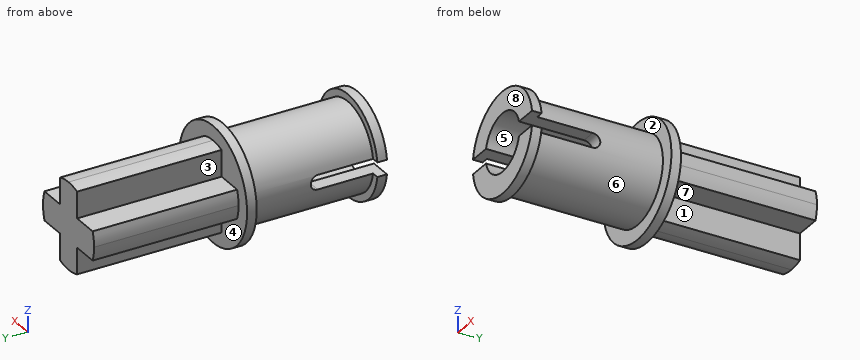
from build123d import *

# Parameters (mm, degrees)
SKETCH1_R               = 1.5
SKETCH1_R_2             = 1
BOSS_EXTRUDE1_DEPTH     = 5
SKETCH2_R               = 2
SKETCH2_R_2             = 1.5
SKETCH2_R_3             = 1
BOSS_EXTRUDE2_DEPTH     = 0.333333333
SKETCH3_R               = 1.75
SKETCH3_R_2             = 1
BOSS_EXTRUDE4_DEPTH     = 0.333333333
SKETCH4_R               = 0.25
SKETCH4_W               = 0.5
SKETCH4_H               = 2.25
CUT_EXTRUDE1_DEPTH      = 6.744562647
CUT_EXTRUDE1_DEPTH_BACK = 6.744562647
SKETCH7_W               = 1
SKETCH7_H               = 1
BOSS_EXTRUDE6_DEPTH     = 5


with BuildPart() as part:
    # Sketch1 → Boss-Extrude1 (new body)
    with BuildSketch(Plane(origin=(0, 0, 0), x_dir=(1, 0, 0), z_dir=(0, 1, 0))):
        with Locations(Location((0, 0, 0), (0, 0, 270))):
            Circle(SKETCH1_R)
        with Locations(Location((0, 0, 0), (0, 0, 270))):
            Circle(SKETCH1_R_2, mode=Mode.SUBTRACT)
    extrude(amount=BOSS_EXTRUDE1_DEPTH)

    # Sketch2 → Boss-Extrude2 (add)
    with BuildSketch(Plane(origin=(0, 5, 0), x_dir=(1, 0, 0), z_dir=(0, 1, 0))):
        with Locations(Location((0, 0, 0), (0, 0, 270))):
            Circle(SKETCH2_R)
        with Locations(Location((0, 0, 0), (0, 0, 270))):
            Circle(SKETCH2_R_2, mode=Mode.SUBTRACT)
        with Locations(Location((0, 0, 0), (0, 0, 270))):
            Circle(SKETCH2_R_2)
        with Locations(Location((0, 0, 0), (0, 0, 270))):
            Circle(SKETCH2_R_3, mode=Mode.SUBTRACT)
        with Locations(Location((0, 0, 0), (0, 0, 270))):
            Circle(SKETCH2_R_3)
    extrude(amount=-BOSS_EXTRUDE2_DEPTH)

    # Sketch3 → Boss-Extrude4 (add)
    with BuildSketch(Plane(origin=(0, 0, 0), x_dir=(-1, 0, 0), z_dir=(0, -1, 0))):
        with Locations(Location((0, 0, 0), (0, 0, 90))):
            Circle(SKETCH3_R)
        with Locations(Location((0, 0, 0), (0, 0, 270))):
            Circle(SKETCH3_R_2, mode=Mode.SUBTRACT)
    extrude(amount=-BOSS_EXTRUDE4_DEPTH)

    # Sketch4 → Cut-Extrude1 (cut, two sides)
    with BuildSketch(Plane(origin=(0, 0, 0), x_dir=(0, 0, -1), z_dir=(1, 0, 0))) as cut_extrude1_sk:
        with Locations((0, 2.25)):
            Circle(SKETCH4_R)
        with Locations((0, 1.125)):
            Rectangle(SKETCH4_W, SKETCH4_H)
    extrude(amount=CUT_EXTRUDE1_DEPTH, mode=Mode.SUBTRACT)
    extrude(cut_extrude1_sk.sketch, amount=-CUT_EXTRUDE1_DEPTH_BACK, mode=Mode.SUBTRACT)

    # Sketch7 → Boss-Extrude6 (add)
    with BuildSketch(Plane(origin=(0, 5, 0), x_dir=(1, 0, 0), z_dir=(0, 1, 0))):
        with BuildLine():
            Line((1.414213562, 0.5), (0.5, 0.5))
            Line((0.5, 0.5), (0.5, -0.5))
            Line((0.5, -0.5), (1.414213562, -0.5))
            ThreePointArc((1.414213562, -0.5), (1.478397839, -0.253652968), (1.5, 0))
            ThreePointArc((1.5, 0), (1.478397839, 0.253652968), (1.414213562, 0.5))
        make_face()
        Rectangle(SKETCH7_W, SKETCH7_H)
        with BuildLine():
            Line((0.5, -0.5), (-0.5, -0.5))
            Line((-0.5, -0.5), (-0.5, -1.414213562))
            ThreePointArc((-0.5, -1.414213562), (-0.253652968, -1.478397839), (0, -1.5))
            ThreePointArc((0, -1.5), (0.253652968, -1.478397839), (0.5, -1.414213562))
            Line((0.5, -1.414213562), (0.5, -0.5))
        make_face()
        with BuildLine():
            ThreePointArc((0.5, 1.414213562), (0.253652968, 1.478397839), (0, 1.5))
            ThreePointArc((0, 1.5), (-0.253652968, 1.478397839), (-0.5, 1.414213562))
            Line((-0.5, 1.414213562), (-0.5, 0.5))
            Line((-0.5, 0.5), (0.5, 0.5))
            Line((0.5, 0.5), (0.5, 1.414213562))
        make_face()
        with BuildLine():
            Line((-0.5, -0.5), (-0.5, 0.5))
            Line((-0.5, 0.5), (-1.414213562, 0.5))
            ThreePointArc((-1.414213562, 0.5), (-1.478397839, 0.253652968), (-1.5, 0))
            ThreePointArc((-1.5, 0), (-1.478397839, -0.253652968), (-1.414213562, -0.5))
            Line((-1.414213562, -0.5), (-0.5, -0.5))
        make_face()
    extrude(amount=BOSS_EXTRUDE6_DEPTH)


solid = part.part
Can you work these out from the model? Positions are in its coordinate system, mm. Face numbers are marked on the shaded views. A direction names the side the tool comes from. Give positions to 0.01 mm unless a question says otherwise; leave off trailing zeros. Order: outer loops, then holes, each group sorted by start corner. A loop starts at its lowest first (then second) coordinate and runs counter-clockwise, first axis right, second up. Notation, with made-up numbers: M 88,46.5 L 128,46.5 A17 cw 128,75.5 Z; hole C -33.5,-40 d6. An arc over 180 degrees is marked long. One line per question, with ' | ' between items.
Item 1: I'm going to push flat-ended pins straight in: pin 1 Ø0.5 at (y, z) = (8.5, -1) entering from +X; pin 2 Ø0.6 at (x, y) = (-1.5, 1) entering from +Z; pin 3 Ø1.5 at (x, y) = (0.5, 9) entering from -Z. Where does each tip first touch, or does it pass through?
Answer block:
pin 1: stops at x = 0.5 | pin 2: stops at z = 0.9 | pin 3: stops at z = -1.5
Item 2: Suppose I cut it at D-D, the plane x = -0.65. Write out the boundary of the cut face in (y, z).
Answer block:
outline: M 0,-1.62 L 0.33,-1.62 L 0.33,-1.35 L 4.67,-1.35 L 4.67,-1.89 L 5,-1.89 L 5,-0.5 L 10,-0.5 L 10,0.5 L 5,0.5 L 5,1.89 L 4.67,1.89 L 4.67,1.35 L 0.33,1.35 L 0.33,1.62 L 0,1.62 L 0,0.76 L 4.67,0.76 L 4.67,-0.76 L 0,-0.76 Z
Item 3: Suppose I cut it at B-B, the plane z = -1.65. Write out the boundary of the cut face in (x, y), then the cut area to 3 significant figures.
Answer block:
outline: M -1.13,4.67 L 1.13,4.67 L 1.13,5 L -1.13,5 Z; M -0.58,0 L 0.58,0 L 0.58,0.33 L -0.58,0.33 Z | area: 1.14 mm2
Item 4: We'd pull the mould along Y, two halves only. Please class the marked faces 6, 7 and 8: released by +Y, released by -Y, zero draft, split by the parting line, or undercut.
Answer block:
face 6: undercut | face 7: zero draft | face 8: released by -Y
Item 5: For the marked faces 1, 2, 3, 4 and 5, which set-ups out of +Z, -Z, +X, -X, +Y, -Y let a thin tool reach every point of the face, with its end or its side?
Answer block:
face 1: -Z, +X, +Y | face 2: none | face 3: +Z, -X, +Y | face 4: +Y | face 5: -Y
Item 6: Please list where these lines run through material, in increasing order: L1, parallel to Z at x = 0, y = 4; L2, parallel to Y at x = 1.5, z = -0.8.
Answer block:
L1: z = -1.5 to -1, 1 to 1.5 | L2: y = 0 to 0.33, 4.67 to 5
Item 7: Suppose I cut it at C-C, the plane y = 5.5. Write out the boundary of the cut face in (x, z), then the cut area to 3 significant figures.
Answer block:
outline: M -1.41,-0.5 L -0.5,-0.5 L -0.5,-1.41 A1.5 ccw 0.5,-1.41 L 0.5,-0.5 L 1.41,-0.5 A1.5 ccw 1.41,0.5 L 0.5,0.5 L 0.5,1.41 A1.5 ccw -0.5,1.41 L -0.5,0.5 L -1.41,0.5 A1.5 ccw Z | area: 4.89 mm2
Item 8: Suppose I cut it at A-A, the plane y = 2. Write out the boundary of the cut face in (x, z), then the cut area to 3 significant figures.
Answer block:
outline: M -1.48,-0.25 A1.5 ccw 1.48,-0.25 L 0.97,-0.25 A1 cw -0.97,-0.25 Z; M -1.48,0.25 L -0.97,0.25 A1 cw 0.97,0.25 L 1.48,0.25 A1.5 ccw Z | area: 3.42 mm2
